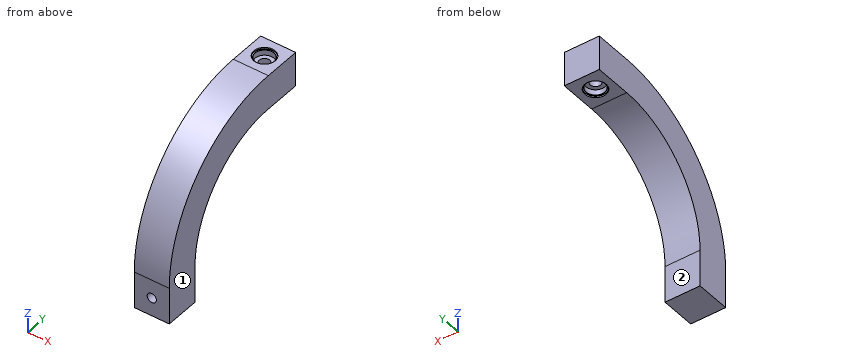
from build123d import *

# Parameters (mm, degrees)
BOSS_EXTRUDE1_DEPTH      = 7.6
BOSS_EXTRUDE1_DEPTH_BACK = 7.6
SKETCH7_R                = 2.25
CUT_EXTRUDE1_DEPTH       = 94.371547498
SKETCH15_R               = 2
CUT_EXTRUDE11_DEPTH      = 10


with BuildPart() as part:
    # Sketch5 → Boss-Extrude1 (new, two sides: drawn at the far end of the back side and taken through both)
    with BuildSketch(Plane(origin=(0, 0, 0), x_dir=(0, 0, -1), z_dir=(1, 0, 0)).offset(-BOSS_EXTRUDE1_DEPTH_BACK)):
        with BuildLine():
            Line((-50.80458146, 8), (-50.80458146, 0))
            Line((-50.80458146, 0), (-50.80458146, -8))
            ThreePointArc((-50.80458146, -8), (-38.267409816, -38.267409816), (-8, -50.80458146))
            Line((-8, -50.80458146), (0, -50.80458146))
            Line((0, -50.80458146), (8, -50.80458146))
            Line((8, -50.80458146), (8, -65.80458146))
            Line((8, -65.80458146), (-8, -65.80458146))
            ThreePointArc((-8, -65.80458146), (-48.874011534, -48.874011534), (-65.80458146, -8))
            Line((-65.80458146, -8), (-65.80458146, 8))
            Line((-65.80458146, 8), (-50.80458146, 8))
        make_face()
    extrude(amount=BOSS_EXTRUDE1_DEPTH + BOSS_EXTRUDE1_DEPTH_BACK)

    # Sketch7 → Cut-Extrude1 (cut, through all)
    with BuildSketch(Plane.XY):
        with Locations(Location((0, 0, 0), (0, 0, 180))):
            Circle(SKETCH7_R)
    extrude(amount=CUT_EXTRUDE1_DEPTH, mode=Mode.SUBTRACT)

    # Sketch15 → Cut-Extrude11 (cut)
    with BuildSketch(Plane.XZ.offset(65.80458146)):
        with Locations(Location((0, 0, 0), (0, 0, 270))):
            Circle(SKETCH15_R)
    extrude(amount=-CUT_EXTRUDE11_DEPTH, mode=Mode.SUBTRACT)

    # Sketch18 → Cut-Revolve1 (revolve, cut)
    with BuildSketch(Plane(origin=(0, 0, 0), x_dir=(0, 0, -1), z_dir=(1, 0, 0)), mode=Mode.PRIVATE) as cut_revolve1_sk:
        with BuildLine():
            Line((-65.80458146, 4.65), (-65.80458146, 0))
            Line((-65.80458146, 0), (-62.80458146, 0))
            Line((-62.80458146, 0), (-62.80458146, 4.05))
            Line((-62.80458146, 4.05), (-65.10458146, 4.05))
            ThreePointArc((-65.10458146, 4.05), (-65.175292138, 4.079289322), (-65.20458146, 4.15))
            Line((-65.20458146, 4.15), (-65.20458146, 4.65))
            Line((-65.20458146, 4.65), (-65.80458146, 4.65))
        make_face()
        with BuildLine():
            Line((-51.40458146, 4.65), (-50.80458146, 4.65))
            Line((-50.80458146, 4.65), (-50.80458146, 0))
            Line((-50.80458146, 0), (-53.80458146, 0))
            Line((-53.80458146, 0), (-53.80458146, 4.05))
            Line((-53.80458146, 4.05), (-51.50458146, 4.05))
            ThreePointArc((-51.50458146, 4.05), (-51.433870782, 4.079289322), (-51.40458146, 4.15))
            Line((-51.40458146, 4.15), (-51.40458146, 4.65))
        make_face()
    revolve(cut_revolve1_sk.sketch.rotate(Axis((0, 0, 109.558527697), (0, 0, -1)), 90), axis=Axis((0, 0, 109.558527697), (0, 0, -1)), mode=Mode.SUBTRACT)


solid = part.part
Could you check a few things on this model? Use its own coordinates, in mm. Face numbers are marked on the shaded views. A direction names the side the tool comes from. Give positions to 0.01 mm unless a question says otherwise; leave off trailing zeros. Loops run counter-clockwise (first coordinate to the right, second up) from the corner with the lowest first, then second, coordinate; pieces in that order, holes last. Notation, with made-up numbers: (30, 22) -> (66, 22) arc R31 cw to (66, 48) -> close; hole circle Ø9 at (20, 33). An arc over 180 degrees is marked (long way). Answer as CSV lines item,"result". Start each with the question number.
(1) I'm going to push flat-ended pins straight in: pin 1 Ø5.5 at (x, y) = (0, 0) entering from -Z; pin 2 Ø8 at (x, y) = (5, -3) entering from -Z; pin 3 Ø1.5 at (x, z) = (-0.5, 40.5) entering from -Y; pin 4 Ø8 at (y, z) = (-42.5, 21) entering from +X. Where does each tip first touch, or does it pass through?
(2) If we section it at B-B on z = 0: Write out the boundary of the cut face in (x, y), then the cut area to 3 significant figures.
(3) If we section it at A-A on y = 0: Write out the boundary of the cut face in (x, z).
(4) If we section it at D-D on y = -22.5: Write out the boundary of the cut face in (x, z), then the cut area to 3 significant figures.
(5) I need wall thicknesses on probe 1 along X at (y, z) = (-61, 0); probe 2 along Z at (x, y) = (2.75, 4); probe 3 along Z at (x, y) = (-1.75, -56). Which ranges of each line are inside material? Lowest first, please.
(6) Which directions (+Z, -Z, +X, -X, +Y, -Y) give clear straight access to the entire face, cutting with the end or side of a thin tool? Please do the marked faces 1 and 2.
(7) If we section it at C-C on x = 6.5: Write out the boundary of the cut face in (y, z).
Computed:
1,pin 1,"stops at z = 53.8"
1,pin 2,"stops at z = 50.8"
1,pin 3,"stops at y = -56.3"
1,pin 4,"passes through"
2,outline,"(-7.6, -65.8) -> (-2, -65.8) -> (-2, -55.8) -> (2, -55.8) -> (2, -65.8) -> (7.6, -65.8) -> (7.6, -50.8) -> (-7.6, -50.8) -> close"
2,area,"188 mm2"
3,outline,"(-7.6, 50.8) -> (-4.65, 50.8) -> (-4.65, 51.4) -> (-4.15, 51.4) arc R0.1 ccw to (-4.05, 51.5) -> (-4.05, 53.8) -> (-2.25, 53.8) -> (-2.25, 62.8) -> (-4.05, 62.8) -> (-4.05, 65.1) arc R0.1 ccw to (-4.15, 65.2) -> (-4.65, 65.2) -> (-4.65, 65.8) -> (-7.6, 65.8) -> close; (2.25, 53.8) -> (4.05, 53.8) -> (4.05, 51.5) arc R0.1 ccw to (4.15, 51.4) -> (4.65, 51.4) -> (4.65, 50.8) -> (7.6, 50.8) -> (7.6, 65.8) -> (4.65, 65.8) -> (4.65, 65.2) -> (4.15, 65.2) arc R0.1 ccw to (4.05, 65.1) -> (4.05, 62.8) -> (2.25, 62.8) -> close"
4,outline,"(-7.6, 48.27) -> (7.6, 48.27) -> (7.6, 63.96) -> (-7.6, 63.96) -> close"
4,area,"238 mm2"
5,probe 1,"x = -7.6 to -2, 2 to 7.6"
5,probe 2,"z = 50.8 to 65.8"
5,probe 3,"z = -8 to -0.97, 0.97 to 40.21"
6,face 1,"+Z, -Z, +X, +Y, -Y"
6,face 2,"-Z, +X, -X, +Y"
7,outline,"(-65.8, -8) -> (-50.8, -8) -> (-50.8, 8) arc R42.8 cw to (-8, 50.8) -> (8, 50.8) -> (8, 65.8) -> (-8, 65.8) arc R57.8 ccw to (-65.8, 8) -> close"
